Can you work these out from the model? Positions are in its coordinate system, mm. Give positions to 0.01 mm unless a question says otherwise; leave off trailing zeros. Order: outer loops, then holes, each group sorted by start corner. A loop starts at its lowest first (then second) coordinate and runs counter-clockwise, first axis right, second up. Notation, with made-up numbers: M 88.25,6 L 143.25,6 A22 ccw 143.25,45 Z; hole C 33.25,3.25 d1. An arc over 180 degrees is marked long. Answer as a JSON object with one key per item and string values.
```python
from build123d import *

# Parameters (mm, degrees)
BOSS_EXTRUDE1_DEPTH        = 3.429
FILLET1_R                  = 1.27
F_1_8_0_1250_DOWEL_HOLE1_D = 3.175


with BuildPart() as part:
    # Sketch2 → Boss-Extrude1 (new body)
    with BuildSketch(Plane.XY):
        with BuildLine():
            Line((-17.292487403, 5.747971587), (-2.159010534, 12.853377269))
            ThreePointArc((-2.159010534, 12.853377269), (0, 13.335), (2.159010534, 12.853377269))
            Line((2.159010534, 12.853377269), (17.292487403, 5.747971587))
            ThreePointArc((17.292487403, 5.747971587), (20.791389907, -1.382548448), (14.593724234, -6.35))
            Line((14.593724234, -6.35), (-14.593724234, -6.35))
            ThreePointArc((-14.593724234, -6.35), (-20.791389907, -1.382548448), (-17.292487403, 5.747971587))
        make_face()
    extrude(amount=BOSS_EXTRUDE1_DEPTH)

    # Fillet1
    fillet1_edges = [part.edges().sort_by_distance(p)[0] for p in [
        (20.791389907, -1.382548448, 3.429),
        (9.725748968, 9.300674428, 3.429),
        (0, 13.335, 3.429),
        (-9.725748968, 9.300674428, 3.429),
        (-20.791389907, -1.382548448, 3.429),
        (0, -6.35, 3.429),
    ]]
    fillet(fillet1_edges, radius=FILLET1_R)

    # 1/8 (0.1250) Dowel Hole1 (through all)
    with Locations(Plane.XY.offset(3.429)):
        with Locations((0, 8.255), (-14.593724234, 0), (14.593724234, 0)):
            Hole(F_1_8_0_1250_DOWEL_HOLE1_D / 2)


solid = part.part
```
1) I need wall thicknesses on L1, parallel to X at y = 7.75, z = 1.25; L2, parallel to X at y = 8.5, z = 1.8; L3, parallel to Y at x = 0.5, z = 1.75. Which ranges of each line are inside material? Lowest first, please.
Results found:
{"L1": "x = -13.03 to -1.51, 1.51 to 13.03", "L2": "x = -11.43 to -1.57, 1.57 to 11.43", "L3": "y = -6.35 to 6.75, 9.76 to 13.31"}
2) I want a section at D-D on z = 2.75. Write out the boundary of the cut face in (x, y) (1 decimal).
Results found:
{"outline": "M -17.2,5.6 A6.2 ccw -14.6,-6.2 L 14.6,-6.2 A6.2 ccw 17.2,5.6 L 2.1,12.7 A4.9 ccw -2.1,12.7 Z; hole C -14.6,0 d3.2; hole C 0,8.3 d3.2; hole C 14.6,0 d3.2"}
3) Thinking about a two-plate mould opening in X: for faces 1 (the face through (16.18, 0.07, 1.69)), 2 (the face through (-13.008, 0.07, 1.69)), 3 (the face through (-9.47, 9.02, 3.05)), 4 (the face through (9.68, 8.92, 3.05)), which applies, pulls with the +X half, pulls with the -X half, needs draft (parallel to the pull), parting line crosses it, or undercut?
Results found:
{"face 1": "undercut", "face 2": "undercut", "face 3": "pulls with the -X half", "face 4": "pulls with the +X half"}
4) I want a section at B-B on z = 0.85. Count the separate pieces of the cut face and the enclosed holes in it, and give its area (3 significant figures).
Results found:
{"separate pieces": "1", "enclosed holes": "3", "area": "593 mm²"}
5) I'm going to push flat-ended pins straight in: pin 1 Ø3 at (x, y) = (-14.59, 0) entering from -Z; pin 2 Ø1 at (y, z) = (-1, 3) entering from -X; pin 3 Ø2 at (x, z) = (16, 1) entering from -Y. Where does each tip first touch, or does it pass through?
Results found:
{"pin 1": "passes through", "pin 2": "stops at x = -20.83", "pin 3": "stops at y = -6.34"}
